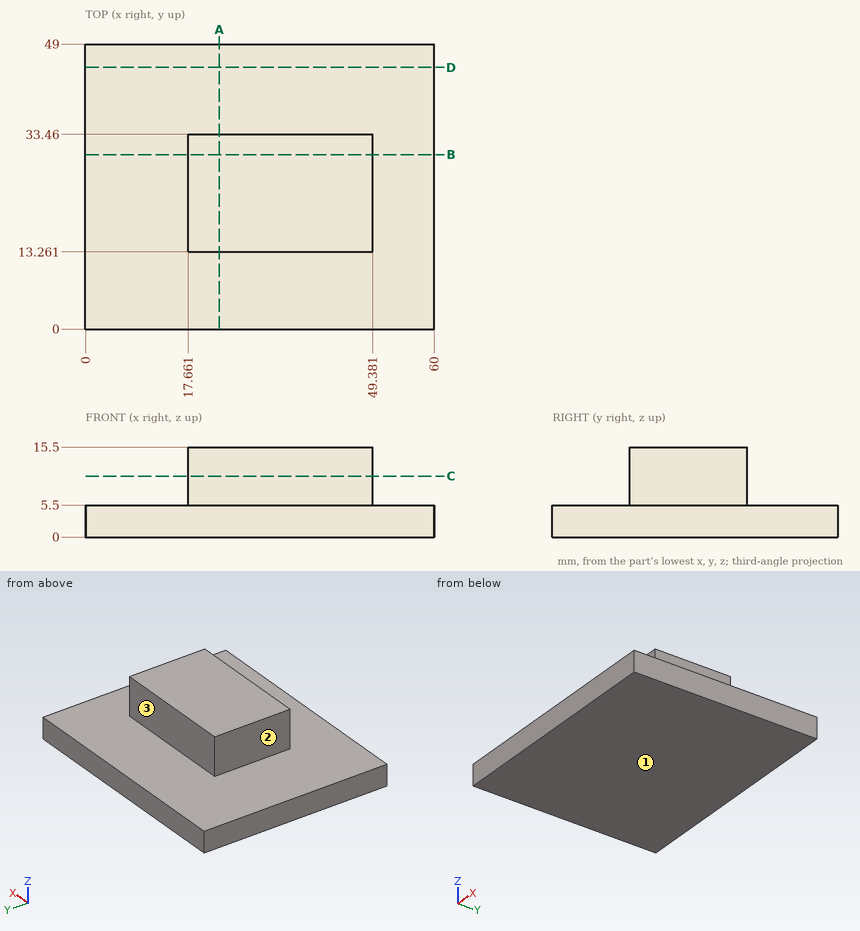
Input: dimensioned drawing with shaded views. Units: mm. Origin: part minimum x, y, z. A direction names the side the tool comes from. Give positions to 0.01 mm unless a question says otherwise; leave off trailing zeros. Write each loop counter-clockwise with the first axis right and the second up, starting at its lowest first coordinate (ties: lowest second). Pieces come first, ordered by that corner, then holes.
1. First-contact query: pin 1 (12 mm diameter, centred on x = 46.5, y = 34, fed in from +Z); pin 2 (8 mm diameter, centred on y = 21.5, z = 13, fed in from -X); pin 3 (8 mm diameter, centred on x = 29.5, z = 11, fed in from -Y). Flat tips, straight axial feed; report the tip coordinate or a pass-through.
2. Section query B-B (y = 30). Return the cut outline in (x, z), then the cut area to 3 significant figures.
3. Access query for the marked faces 1, 2 and 3. Directions: +Z, -Z, +X, -X, +Y, -Y. A direction counts if a zero-diameter tool reaches every point of the face in a straight line with its end or side. Return the directions, or none.
4. Material intervals for line 1 along Y through (x, z) = (23, 12.25); line 2 along Z through (x, y) = (26, 5.5); line 3 along X through (y, z) = (29.5, 10), sorted ascending.
5. Section query A-A (x = 23). Return the cut outline in (y, z).
6. Section query D-D (y = 45). Return the cut outline in (x, z), then the cut area to 3 significant figures.
7. Section query C-C (z = 10.5). Return the cut outline in (x, y).
Output values:
1. pin 1: stops at z = 15.5
1. pin 2: stops at x = 17.66
1. pin 3: stops at y = 13.26
2. outline: (0, 0) - (60, 0) - (60, 5.5) - (49.38, 5.5) - (49.38, 15.5) - (17.66, 15.5) - (17.66, 5.5) - (0, 5.5) - close
2. area: 647 mm2
3. face 1: -Z, +X, -X, +Y, -Y
3. face 2: +Z, -X, +Y, -Y
3. face 3: +Z, +X, -X, +Y
4. line 1: y = 13.26 to 33.46
4. line 2: z = 0 to 5.5
4. line 3: x = 17.66 to 49.38
5. outline: (0, 0) - (49, 0) - (49, 5.5) - (33.46, 5.5) - (33.46, 15.5) - (13.26, 15.5) - (13.26, 5.5) - (0, 5.5) - close
6. outline: (0, 0) - (60, 0) - (60, 5.5) - (0, 5.5) - close
6. area: 330 mm2
7. outline: (17.66, 13.26) - (49.38, 13.26) - (49.38, 33.46) - (17.66, 33.46) - close
